from build123d import *

# Parameters (mm, degrees)
SKETCH1_R               = 2
BOSS_EXTRUDE1_DEPTH     = 5
SKETCH3_R               = 12.5
SKETCH3_W               = 5
SKETCH3_H               = 10
CUT_EXTRUDE5_DEPTH      = 1
CUT_EXTRUDE5_DEPTH_BACK = 6


with BuildPart() as part:
    # Sketch1 → Boss-Extrude1 (new body)
    with BuildSketch(Plane.XY):
        Polygon((2.5, -200), (2.5, 0), (-2.5, 0), (-30.5, 0), (-203.705080757, -100), (-30.5, -200), align=None)
        with Locations((-37.5, -30)):
            Circle(SKETCH1_R, mode=Mode.SUBTRACT)
        with Locations((-27.5, -30)):
            Circle(SKETCH1_R, mode=Mode.SUBTRACT)
        with Locations((-17.5, -30)):
            Circle(SKETCH1_R, mode=Mode.SUBTRACT)
        with Locations((-37.5, -20)):
            Circle(SKETCH1_R, mode=Mode.SUBTRACT)
        with Locations((-27.5, -20)):
            Circle(SKETCH1_R, mode=Mode.SUBTRACT)
        with Locations((-17.5, -20)):
            Circle(SKETCH1_R, mode=Mode.SUBTRACT)
    extrude(amount=BOSS_EXTRUDE1_DEPTH)

    # Sketch3 → Cut-Extrude5 (cut, two sides)
    with BuildSketch(Plane.XY.offset(5)) as cut_extrude5_sk:
        with Locations((-88.235026919, -100)):
            Circle(SKETCH3_R)
        Polygon((-121.432667397, -52.5), (-112.77241336, -47.5), (-110.27241336, -51.830127019), (-118.932667397, -56.830127019), align=None)
        Polygon((-101.612159322, -46.830127019), (-104.112159322, -42.5), (-95.451905284, -37.5), (-92.951905284, -41.830127019), align=None)
        Polygon((-84.291651246, -36.830127019), (-86.791651246, -32.5), (-78.131397208, -27.5), (-75.631397208, -31.830127019), align=None)
        Polygon((-66.97114317, -26.830127019), (-69.47114317, -22.5), (-60.810889132, -17.5), (-58.310889132, -21.830127019), align=None)
        Polygon((-49.650635095, -16.830127019), (-52.150635095, -12.5), (-43.490381057, -7.5), (-40.990381057, -11.830127019), align=None)
        Polygon((-136.253175473, -66.830127019), (-138.753175473, -62.5), (-130.092921435, -57.5), (-127.592921435, -61.830127019), align=None)
        Polygon((-153.573683549, -76.830127019), (-156.073683549, -72.5), (-147.413429511, -67.5), (-144.913429511, -71.830127019), align=None)
        Polygon((-170.894191624, -86.830127019), (-173.394191624, -82.5), (-164.733937587, -77.5), (-162.233937587, -81.830127019), align=None)
        Polygon((-112.77241336, -152.5), (-110.27241336, -148.169872981), (-118.932667397, -143.169872981), (-121.432667397, -147.5), align=None)
        Polygon((-173.394191624, -117.5), (-164.733937587, -122.5), (-162.233937587, -118.169872981), (-170.894191624, -113.169872981), align=None)
        Polygon((-156.073683549, -127.5), (-147.413429511, -132.5), (-144.913429511, -128.169872981), (-153.573683549, -123.169872981), align=None)
        Polygon((-138.753175473, -137.5), (-130.092921435, -142.5), (-127.592921435, -138.169872981), (-136.253175473, -133.169872981), align=None)
        Polygon((-52.150635095, -187.5), (-43.490381057, -192.5), (-40.990381057, -188.169872981), (-49.650635095, -183.169872981), align=None)
        Polygon((-69.47114317, -177.5), (-60.810889132, -182.5), (-58.310889132, -178.169872981), (-66.97114317, -173.169872981), align=None)
        Polygon((-86.791651246, -167.5), (-78.131397208, -172.5), (-75.631397208, -168.169872981), (-84.291651246, -163.169872981), align=None)
        Polygon((-104.112159322, -157.5), (-95.451905284, -162.5), (-92.951905284, -158.169872981), (-101.612159322, -153.169872981), align=None)
        with Locations((0, -85)):
            Rectangle(SKETCH3_W, SKETCH3_H)
        with Locations((0, -105)):
            Rectangle(SKETCH3_W, SKETCH3_H)
        with Locations((0, -65)):
            Rectangle(SKETCH3_W, SKETCH3_H)
        with Locations((0, -45)):
            Rectangle(SKETCH3_W, SKETCH3_H)
        with Locations((0, -25)):
            Rectangle(SKETCH3_W, SKETCH3_H)
        with Locations((0, -125)):
            Rectangle(SKETCH3_W, SKETCH3_H)
        with Locations((0, -145)):
            Rectangle(SKETCH3_W, SKETCH3_H)
        with Locations((0, -165)):
            Rectangle(SKETCH3_W, SKETCH3_H)
        with Locations((0, -185)):
            Rectangle(SKETCH3_W, SKETCH3_H)
    extrude(amount=CUT_EXTRUDE5_DEPTH, mode=Mode.SUBTRACT)
    extrude(cut_extrude5_sk.sketch, amount=-CUT_EXTRUDE5_DEPTH_BACK, mode=Mode.SUBTRACT)


solid = part.part
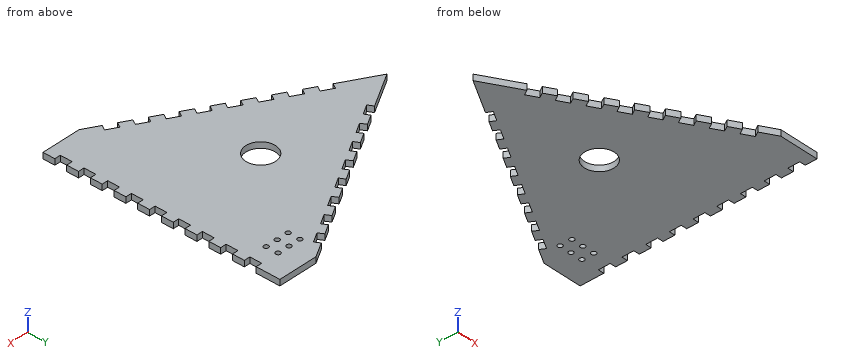
Check sheet for the modelled part. Datum: model origin and axes. Units: mm. Give positions to 0.01 mm unless a question says otherwise; leave off trailing zeros. Answer as CSV lines item,"result".
1. Go/stop test with flat-tipped pins: P1, Ø3, axis at x = -67.5, y = -20.5, coming from the +Z side; P2, Ø1.5, axis at y = -103.5, z = 1.5, coming from the +X side; P3, Ø1.5, axis at x = -169, z = 4.5, coming from the -Y side; P4, Ø1, axis at x = -107.5, z = 4, coming from the -Y side. Record where each tip stops, or that it passes through.
Result sheet:
P1,"through"
P2,"x = -2.5"
P3,"y = -114.7"
P4,"y = -155.83"
2. Scan lines: probe 1 along Y at (x, z) = (-27.5, 1.7); probe 2 along Y at (x, z) = (-37.5, 2.25); probe 3 along X at (y, z) = (-154, 4.4). Record each from-to range of solid material in increasing order. Write a range as from..to.
Result sheet:
probe 1,"-200..-32, -28..-22, -18..0"
probe 2,"-195.96..-32, -28..-22, -18..-4.04"
probe 3,"-110.17..-102.09, -100.17..2.5"
3. Section check A-A (z = 2.5). State how many separate pieces and enclosed holes the cut face has, then the cut area to 3 significant figures.
Result sheet:
separate pieces,"1"
enclosed holes,"7"
area,"22,100 mm²"
